Print and shaded views of the part. All mm, measured from the part's lowest x, y and z. Coordinates: 2 decimals unless noted, no trailing zeros. Order: outer loops, then holes, each group sorted by start corner. A loop starts at its lowest first (then second) coordinate and runs counter-clockwise, first axis right, second up. Notation, with made-up numbers: (36.5, 67.5) - (79.5, 67.5) arc R27 ccw to (79.5, 99.5) - close; hole circle Ø4 at (28.25, 81). An arc over 180 degrees is marked (long way). Write each question's results on one line, items separated by ' | '.
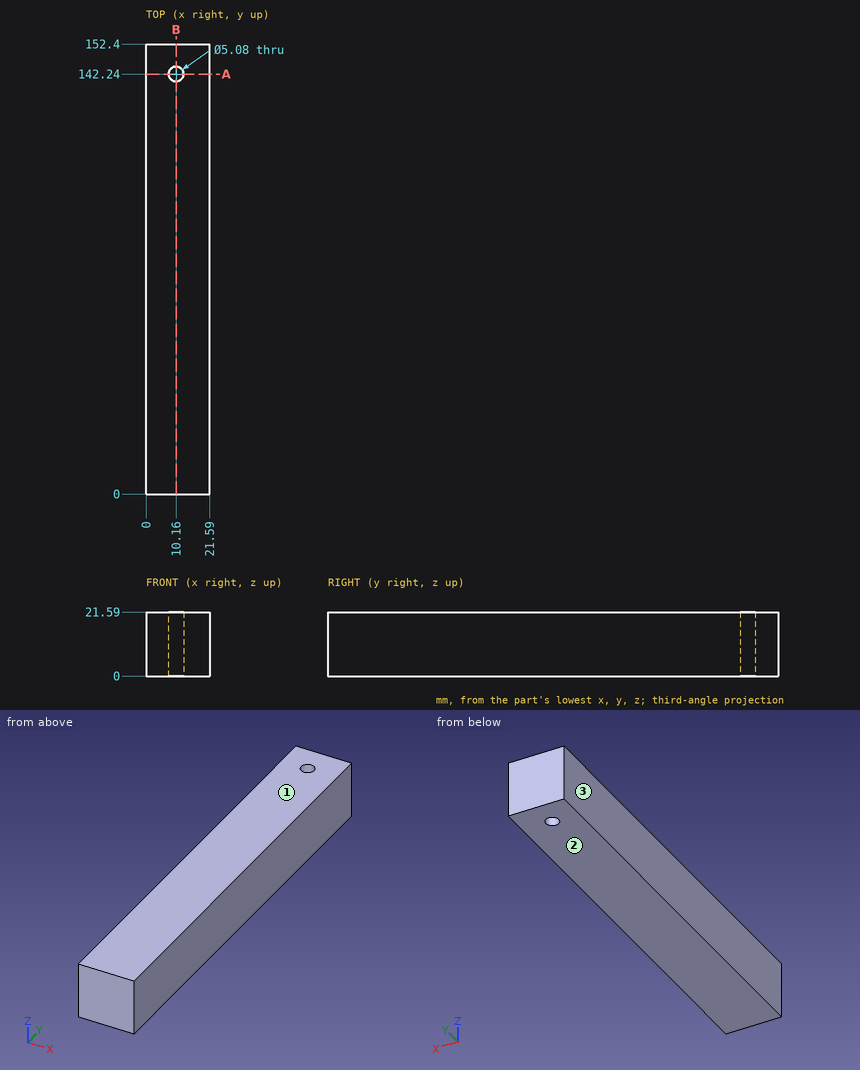
1. Band-saw the part on A-A on y = 142.24. Give the cut face in (x, z).
Solved:
outline: (0, 0) - (7.62, 0) - (7.62, 21.59) - (0, 21.59) - close; (12.7, 0) - (21.59, 0) - (21.59, 21.59) - (12.7, 21.59) - close
2. Band-saw the part on B-B on x = 10.16. Give the cut face in (y, z).
Solved:
outline: (0, 0) - (139.7, 0) - (139.7, 21.59) - (0, 21.59) - close; (144.78, 0) - (152.4, 0) - (152.4, 21.59) - (144.78, 21.59) - close
3. Two-plate mould, pull along Z, no slides. Class the marked faces 1, 2 and 3: +Z half, -Z half, draft (parallel to the pull), parting line (faces both ways), or undercut.
Solved:
face 1: +Z half | face 2: -Z half | face 3: draft
4. Drop a flat-ended pin along its axis: pin 1 Ø4 at (x, y) = (10.16, 142.24) entering from +Z. Give the stop position or say it passes through.
Solved:
pin 1: passes through
5. Probe line 1 (Y direction, x = 10.16, z = 13.5); line 2 (X direction, y = 142.24, z = 13.5); line 3 (Y direction, x = 8.5, z = 13.5). List the from-to ranges inside material, lowest first.
Solved:
line 1: y = 0 to 139.7, 144.78 to 152.4 | line 2: x = 0 to 7.62, 12.7 to 21.59 | line 3: y = 0 to 140.32, 144.16 to 152.4
